Build history of the part. All positions in model axes, mm. Face numbers are marked on the shaded views. A direction names the side the tool comes from. Round coordinates to 2 decimals unless told otherwise and drop trailing zeros. Write each loop counter-clockwise with the first axis right and the second up, starting at its lowest first coordinate (ties: lowest second). Pieces come first, ordered by that corner, then holes. Notation, with made-up numbers: (83.25, 87.5) -> (104.25, 87.5) arc R26 ccw to (104.25, 108.5) -> close; hole circle Ø9 at (-2, 19.5). An arc over 180 degrees is marked (long way). Answer in a Markdown table with one row per item.
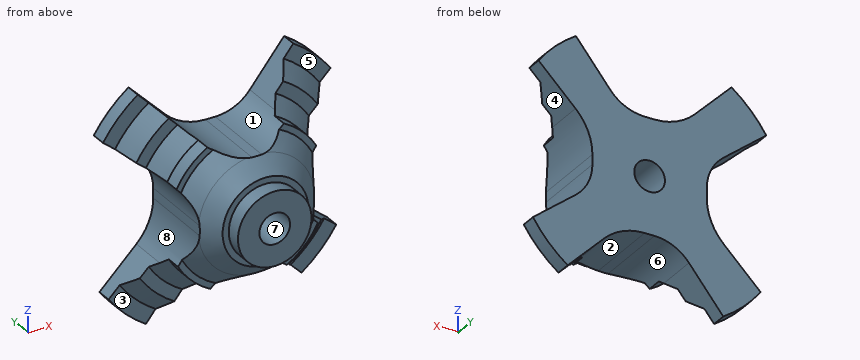
```python
from build123d import *

# Parameters (mm, degrees)
F0_R      = 12
F0_R_2    = 5
F1_DEPTH  = 35
F0_R_3    = 19
F2_DEPTH  = 30
F0_R_4    = 26
F3_DEPTH  = 20
F0_R_5    = 40
F4_DEPTH  = 10
F0_R_6    = 45
F5_DEPTH  = 5
F9_SIZE   = 4.99999
F10_DEPTH = 50
F11_SIZE  = 4.99999
F13_DEPTH = 50
F14_R     = 18.5105769834
F15_R     = 14.4105910726
F16_ANGLE = 90
F17_ANGLE = 180
F18_ANGLE = 270


# Not quite as in the source:
# - a fillet or chamfer is up to 0.001 mm smaller than in the source, because OpenCascade refuses the exact size


with BuildPart() as f1:
    # F0 (on Front) → F1 (new body)
    with BuildSketch(Plane.XZ):
        Circle(F0_R)
        Circle(F0_R_2, mode=Mode.SUBTRACT)
    extrude(amount=F1_DEPTH)

    # F0 (on Front) → F2 (join)
    with BuildSketch(Plane.XZ):
        Circle(F0_R_3)
        Circle(F0_R, mode=Mode.SUBTRACT)
    extrude(amount=F2_DEPTH)

    # F0 (on Front) → F3 (join)
    with BuildSketch(Plane.XZ):
        Circle(F0_R_4)
        Circle(F0_R_3, mode=Mode.SUBTRACT)
    extrude(amount=F3_DEPTH)

    # F0 (on Front) → F4 (join)
    with BuildSketch(Plane.XZ):
        Circle(F0_R_5)
        Circle(F0_R_4, mode=Mode.SUBTRACT)
    extrude(amount=F4_DEPTH)

    # F0 (on Front) → F5 (join)
    with BuildSketch(Plane.XZ):
        Circle(F0_R_6)
        Circle(F0_R_5, mode=Mode.SUBTRACT)
    extrude(amount=F5_DEPTH)

    # F9 (size 5 in the source; OpenCascade refuses exactly that, so slightly less here)
    f9_edges = [f1.edges().sort_by_distance(p)[0] for p in [
        (-40, -10, 0),
        (-26, -10, 0),
    ]]
    chamfer(f9_edges, length=F9_SIZE)

    # F0 (on Front) → F10 (cut)
    with BuildSketch(Plane.XZ):
        Circle(F0_R_2)
    extrude(amount=-F10_DEPTH, mode=Mode.SUBTRACT)

    # F11 (size 5 in the source; OpenCascade refuses exactly that, so slightly less here)
    f11_edges = [f1.edges().sort_by_distance(p)[0] for p in [
        (-19, -20, 0),
        (19, -25, 0),
        (-19, -30, 0),
    ]]
    chamfer(f11_edges, length=F11_SIZE)


with BuildPart() as f13:
    # F12 (on Front) → F13 (new body)
    with BuildSketch(Plane.XZ):
        Polygon((30.8662448078, 46.592772007), (-38.6121459305, 48.2358410954), (-9.3319928274, 18.6549890786), (8.5259051993, 18.6549890786), align=None)
    extrude(amount=F13_DEPTH)

    # F14
    f14_edges = [f13.edges().sort_by_distance(p)[0] for p in [
        (-9.331993, -25, 18.654989),
    ]]
    fillet(f14_edges, radius=F14_R)

    # F15
    f15_edges = [f13.edges().sort_by_distance(p)[0] for p in [
        (8.525905, -25, 18.654989),
    ]]
    fillet(f15_edges, radius=F15_R)


with BuildPart() as f16_1:
    # F16: copy of F13
    add(f13.part.rotate(Axis((0, -35.1110678166, 0), (0, 1, 0)), F16_ANGLE))


with BuildPart() as f17_1:
    # F17: copy of F13
    add(f13.part.rotate(Axis((0, -20.7477975637, 0), (0, 1, 0)), F17_ANGLE))


with BuildPart() as f18_1:
    # F18: copy of F13
    add(f13.part.rotate(Axis((0, -17.8390480578, 0), (0, 1, 0)), F18_ANGLE))


with BuildPart() as f1_1:
    add(f1.part)

    # F19: cut F13
    add(f13.part, mode=Mode.SUBTRACT)

    # F20: cut F17_1
    add(f17_1.part, mode=Mode.SUBTRACT)

    # F21: cut F16_1
    add(f16_1.part, mode=Mode.SUBTRACT)

    # F22: cut F18_1
    add(f18_1.part, mode=Mode.SUBTRACT)


solid = f1_1.part
```
Q1. Which spindle directions (+Z, -Z, +X, -X, +Y, -Y) get a long thin tool onto all of the face, cutting with end or side? Do the marked faces 1, 2, 3 and 4. Say none if no direction does.
A:
| item | result |
|---|---|
| face 1 | +Z, +Y, -Y |
| face 2 | -Z, +Y, -Y |
| face 3 | -Z, -X, -Y |
| face 4 | +X, +Y, -Y |
Q2. Drop flat-ended pins along their axis: P1, Ø15, axis at x = 25, z = -25, coming from the -Y side; P2, Ø6, axis at x = -18.5, z = 10.5, coming from the -Y side; P3, Ø5, axis at x = -15, y = -11.5, coming from the +Z side; P4, Ø3, axis at x = -11, z = -14, coming from the +Y side. Give the stop position or say it passes through.
A:
| item | result |
|---|---|
| P1 | y = -13.14 |
| P2 | y = -25.73 |
| P3 | z = 26.4 |
| P4 | y = 0 |
Q3. Wall check: line 1 (Z direction, x = 0, y = -14.5); line 2 (X direction, y = -12.5, z = 2); line 3 (Y direction, x = -6.5, z = 11.5). Give the ranges that are in metal, low to high. Write a range as [from, to].
A:
| item | result |
|---|---|
| line 1 | [-18.65, -5], [5, 18.65] |
| line 2 | [-18.66, -4.58], [4.58, 18.66] |
| line 3 | [-30, 0] |
Q4. Saw through at A-A on x = 0. Write the cut outline in (y, z), plus the area to 3 significant figures.
A:
| item | result |
|---|---|
| outline | (-35, -12) -> (-30, -12) -> (-30, -14) -> (-25.35, -18.65) -> (0, -18.65) -> (0, -5) -> (-35, -5) -> close; (-35, 5) -> (0, 5) -> (0, 18.65) -> (-25.35, 18.65) -> (-30, 14) -> (-30, 12) -> (-35, 12) -> close |
| area | 868 mm² |
Q5. Saw through at C-C on y = -22. Write the cut outline in (x, z), plus the area to 3 significant figures.
A:
| item | result |
|---|---|
| outline | (-20.35, 8.37) arc R14.41 cw to (-18.65, 1.6) -> (-18.65, -1.61) arc R18.51 cw to (-20.14, -8.86) arc R22 ccw to (-8.37, -20.35) arc R14.41 cw to (-1.6, -18.65) -> (1.61, -18.65) arc R18.51 cw to (8.86, -20.14) arc R22 ccw to (20.35, -8.37) arc R14.41 cw to (18.65, -1.6) -> (18.65, 1.61) arc R18.51 cw to (20.14, 8.86) arc R22 ccw to (8.37, 20.35) arc R14.41 cw to (1.6, 18.65) -> (-1.61, 18.65) arc R18.51 cw to (-8.86, 20.14) arc R22 ccw to start; hole circle Ø10 at (0, 0) |
| area | 1,280 mm² |
Q6. Saw through at B-B on z = 0. Write the cut outline in (x, y), plus the area to 3 significant figures.
A:
| item | result |
|---|---|
| outline | (-18.65, -25.35) -> (-14, -30) -> (-12, -30) -> (-12, -35) -> (-5, -35) -> (-5, 0) -> (-18.65, 0) -> close; (5, -35) -> (12, -35) -> (12, -30) -> (14, -30) -> (18.65, -25.35) -> (18.65, 0) -> (5, 0) -> close |
| area | 868 mm² |
Q7. Two-plate mould, pull along Z, no slides. Class the marked faces 5, 6, 7 and 8: released by +Z, released by -Z, zero draft, split by the parting line, or undercut.
A:
| item | result |
|---|---|
| face 5 | zero draft |
| face 6 | released by -Z |
| face 7 | undercut |
| face 8 | undercut |
